Work out the finished part from the listing and answer in its coordinate system (mm). Face numbers are marked on the shaded views. Round coordinates to 2 decimals unless told otherwise and drop trailing zeros. Put each result on its own line as item: value.
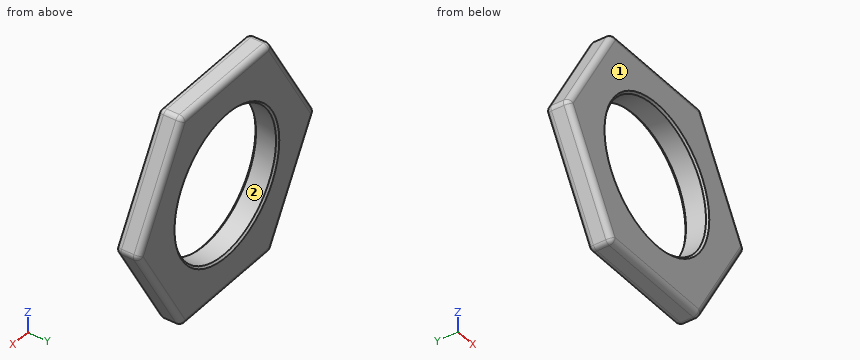
```python
from build123d import *

# Parameters (mm, degrees)
SKETCH1_R           = 9.525
BOSS_EXTRUDE1_DEPTH = 3.175
CHAMFER1_SIZE       = 0.254
FILLET1_R           = 0.762


with BuildPart() as part:
    # Sketch1 → Boss-Extrude1 (new body)
    with BuildSketch(Plane(origin=(0, 0, 0), x_dir=(1, 0, 0), z_dir=(0, 1, 0))):
        Polygon((-8.248891971, -14.2875), (8.248891971, -14.2875), (16.497783942, 0), (8.248891971, 14.2875), (-8.248891971, 14.2875), (-16.497783942, 0), align=None)
        Circle(SKETCH1_R, mode=Mode.SUBTRACT)
    extrude(amount=BOSS_EXTRUDE1_DEPTH)

    # Chamfer1
    chamfer1_edges = [part.edges().sort_by_distance(p)[0] for p in [
        (-9.525, 0, 0),
        (-9.525, 3.175, 0),
    ]]
    chamfer(chamfer1_edges, length=CHAMFER1_SIZE)

    # Fillet1
    fillet1_edges = [part.edges().sort_by_distance(p)[0] for p in [
        (12.373337957, 3.175, 7.14375),
        (-16.497783942, 1.5875, 0),
        (-8.248891971, 1.5875, -14.2875),
        (8.248891971, 1.5875, -14.2875),
        (16.497783942, 1.5875, 0),
        (8.248891971, 1.5875, 14.2875),
        (-8.248891971, 1.5875, 14.2875),
        (12.373337957, 3.175, -7.14375),
        (0, 3.175, -14.2875),
        (-12.373337957, 3.175, -7.14375),
        (-12.373337957, 3.175, 7.14375),
        (-12.373337957, 0, -7.14375),
        (0, 0, -14.2875),
        (12.373337957, 0, -7.14375),
        (0, 3.175, 14.2875),
        (12.373337957, 0, 7.14375),
        (0, 0, 14.2875),
        (-12.373337957, 0, 7.14375),
    ]]
    fillet(fillet1_edges, radius=FILLET1_R)


solid = part.part
```
1) Given pin 1 Ø12 at (x, z) = (-7, -3.5) entering from -Y, flat-ended and moving along its own axis, determine where the tip first touches the part or whether it passes through.
Findings below:
pin 1: stops at y = 0
2) Straight lines are drawn through the part: L1, parallel to Z at x = 0, y = 1 (1 decimal); L2, parallel to X at y = 0.8, z = 0 (3 decimals); L3, parallel to X at y = 2.9, z = 1. For each, find the intervals that lie inside material, in ascending order. Write a range as from..to.
Findings below:
L1: z = -14.3..-9.5, 9.5..14.3
L2: x = -16.38..-9.525, 9.525..16.38
L3: x = -15.72..-9.47, 9.47..15.72
3) For a pull along Z with two mould halves and no side action, classify the marked faces 1 and 2 as pulls with the +Z half, pulls with the -Z half, needs draft (parallel to the pull), parting line crosses it, or undercut.
Findings below:
face 1: needs draft
face 2: undercut
